Source: CAD feature listing. Evaluate the final solid. Frame: model axes, mm. Coordinates: 2 decimals unless noted, no trailing zeros. Order: outer loops, then holes, each group sorted by start corner. A loop starts at its lowest first (then second) coordinate and runs counter-clockwise, first axis right, second up.
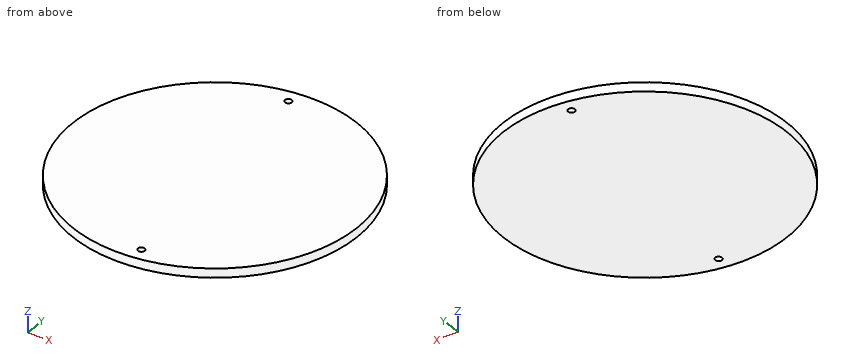
```python
from build123d import *

# Parameters (mm, degrees)
F0_R     = 62.5
F1_DEPTH = 4
F2_R     = 1.5
F3_DEPTH = 4.001
F4_R     = 1.5
F5_DEPTH = 4.001


with BuildPart() as f1:
    # F0 (on Top) → F1 (new body)
    with BuildSketch(Plane.XY):
        Circle(F0_R)
    extrude(amount=F1_DEPTH)

    # F2 (on face) → F3 (cut, through all)
    with BuildSketch(Plane.XY.offset(4)):
        with Locations((-5.9, 56.191102)):
            Circle(F2_R)
    extrude(amount=-F3_DEPTH, mode=Mode.SUBTRACT)

    # F4 (on face) → F5 (cut, through all)
    with BuildSketch(Plane.XY.offset(4)):
        with Locations((5.9, -56.191102)):
            Circle(F4_R)
    extrude(amount=-F5_DEPTH, mode=Mode.SUBTRACT)


solid = f1.part
```
1. Section query A-A on x = -5.9. Return loops of the section in (y, z), plus the area to 3 significant figures.
Findings:
outline: (-62.22, 0) - (54.69, 0) - (54.69, 4) - (-62.22, 4) - close; (57.69, 0) - (62.22, 0) - (62.22, 4) - (57.69, 4) - close
area: 486 mm2
2. Pin query (flat end, axial travel): P1, Ø2.5, axis at x = -5.9, y = 56.19, coming from the +Z side; P2, Ø1.5, axis at x = -9.5, z = 2, coming from the -Y side; P3, Ø2, axis at y = 33.5, z = 3.5, coming from the +X side. Return the tip coordinate at first contact, or that it passes through.
Findings:
P1: passes through
P2: stops at y = -61.88
P3: stops at x = 53.39
3. Section query C-C on x = 16. Return loops of the section in (y, z).
Findings:
outline: (-60.42, 0) - (60.42, 0) - (60.42, 4) - (-60.42, 4) - close
4. Section query B-B on z = 2.8. Return loops of the section in (x, y), plus the area to 3 significant figures.
Findings:
outline: circle Ø125 at (0, 0); hole circle Ø3 at (-5.9, 56.19); hole circle Ø3 at (5.9, -56.19)
area: 12,300 mm2
5. Section query D-D on y = -31. Return loops of the section in (x, z).
Findings:
outline: (-54.27, 0) - (54.27, 0) - (54.27, 4) - (-54.27, 4) - close
6. Ray query, line 1 (Y direction, x = 5.9, z = 1.55); line 2 (X direction, y = 55, z = 2.1); line 3 (Y direction, x = -18.5, z = 3.55). Return the intervals inside material, ascending.
Findings:
line 1: y = -62.22 to -57.69, -54.69 to 62.22
line 2: x = -29.69 to -6.81, -4.99 to 29.69
line 3: y = -59.7 to 59.7
